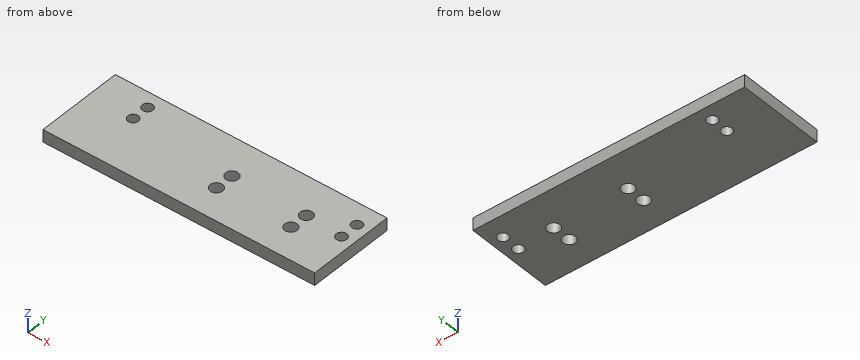
Autodesk Inventor part; units mm, degrees
ref_plane "YZ Plane" through (0, 0, 0) normal (1, 0, 0) x (0, 1, 0)
ref_plane "XZ Plane" through (0, 0, 0) normal (0, 1, 0) x (-1, 0, 0)
ref_plane "XY Plane" through (0, 0, 0) normal (0, 0, 1) x (1, 0, 0)
sketch "Sketch1" plane through (0, 0, 0) normal (0, 0, 1) x (1, 0, 0)
  line L0 (-109.5, 50) -> (109.5, 50)
  line L1 (109.5, 50) -> (-109.5, 50)
  line L2 (-109.5, 50) -> (-109.5, -20)
  line L3 (-109.5, -20) -> (109.5, -20)
  line L4 (109.5, -20) -> (109.5, 50)
  dimension "d81" = 219
  dimension "d82" = 70
  dimension "d83" = 90
  dimension "d84" = 219
extrude "Extrusion1" add sketch "Sketch1" along normal blind 10
sketch "Sketch7" plane through (0, 0, 10) normal (0, 0, 1) x (1, 0, 0)
  line L0 (109.5, -50) -> (109.5, 50)
  line L1 (109.5, 50) -> (109.5, 18)
  line L2 (109.5, 18) -> (99.5, 18)
  line L3 (109.5, 50) -> (87.5, 50)
  line L4 (99.5, 50) -> (99.5, 33)
  line L5 (-109.5, 50) -> (-109.5, -50)
  line L6 (-109.5, 50) -> (-73.5, 50) construction
  line L7 (109.5, 50) -> (-109.5, 50)
  line L8 (-109.5, 50) -> (-73.5, 50)
  line L9 (-73.5, 50) -> (-73.5, 38)
  line L10 (-73.5, 38) -> (-73.5, 24)
  line L11 (87.5, 50) -> (87.5, -50)
  dimension "d32" = 32
  dimension "d34" = 10
  dimension "d36" = 17
  dimension "d37" = 10
  dimension "d41" = 36
  dimension "d42" = 12
  dimension "d43" = 14
hole "Hole1" at (99.5, 33, 10) at (99.5, 18, 10) at (-73.5, 24, 10) at (-73.5, 38, 10) direction (0, 0, -1) diameter 8.5 end through all
sketch "Sketch8" plane through (0, 0, 10) normal (0, 0, 1) x (1, 0, 0)
  line L0 (109.5, -50) -> (109.5, 50)
  line L1 (109.5, 50) -> (109.5, 20)
  line L2 (109.5, 20) -> (109.5, 5)
  line L3 (109.5, 5) -> (69.5, 5)
  line L4 (69.5, 5) -> (9.5, 5)
  line L5 (9.5, 5) -> (9.5, 20)
  line L6 (69.5, 5) -> (69.5, 20)
  point P0 (0, 0)
  dimension "d58" = 30
  dimension "d59" = 15
  dimension "d60" = 40
  dimension "d61" = 60
  dimension "d62" = 15
  dimension "d70" = 15
hole "Hole2" at (9.5, 5, 10) at (9.5, 20, 10) at (69.5, 5, 10) at (69.5, 20, 10) direction (0, 0, -1) diameter 10 end through all
thread "Thread1"
thread "Thread2"
thread "Thread3"
thread "Thread4"
equation "\"d49\" = Thickness"
equation "\"d68\" = Thickness"
equation "\"BendRadius\" = Thickness"
equation "\"BendReliefWidth\" = Thickness"
equation "\"BendReliefDepth\" = 0.5 * Thickness"
equation "\"CornerReliefSize\" = 4 * Thickness"
equation "\"MinimumRemnant\" = 2 * Thickness"
equation "\"TransitionRadius\" = BendRadius"
equation "\"JacobiRadiusSize\" = Thickness"
equation "\"GapSize\" = Thickness"
properties part number "Ball screw right hand support" material "Steel"
Design review of the part built by this model. Coordinates are the model's own, in mm. Round coordinates to 2 decimals unless told otherwise and drop trailing zeros. Order: outer loops, then holes, each group sorted by start corner. A loop starts at its lowest first (then second) coordinate and runs counter-clockwise, first axis right, second up.
1) For L1, parallel to Y at x = 99.5, z = 5.75; L2, parallel to Y at x = 9.5, z = 3.5; L3, parallel to X at y = 4.5, z = 3, list the stretches that pass through material, from the lowest coordinate up.
The answers:
L1: y = -20 to 13.75, 22.25 to 28.75, 37.25 to 50
L2: y = -20 to 0, 10 to 15, 25 to 50
L3: x = -109.5 to 4.53, 14.47 to 64.53, 74.47 to 109.5
2) Consider section C-C (z = 2.75). Count the separate pieces of the cut face and the enclosed holes in it, plus the area to 3 significant figures.
The answers:
separate pieces: 1
enclosed holes: 8
area: 14,800 mm2
3) Consider section B-B (y = 5). State the section outline as (x, z) points, plus the area to 3 significant figures.
The answers:
outline: (-109.5, 0) - (4.5, 0) - (4.5, 10) - (-109.5, 10) - close; (14.5, 0) - (64.5, 0) - (64.5, 10) - (14.5, 10) - close; (74.5, 0) - (109.5, 0) - (109.5, 10) - (74.5, 10) - close
area: 1,990 mm2
4) Consider section A-A (x = 9.5). State the section outline as (y, z) points.
The answers:
outline: (-20, 0) - (0, 0) - (0, 10) - (-20, 10) - close; (10, 0) - (15, 0) - (15, 10) - (10, 10) - close; (25, 0) - (50, 0) - (50, 10) - (25, 10) - close
